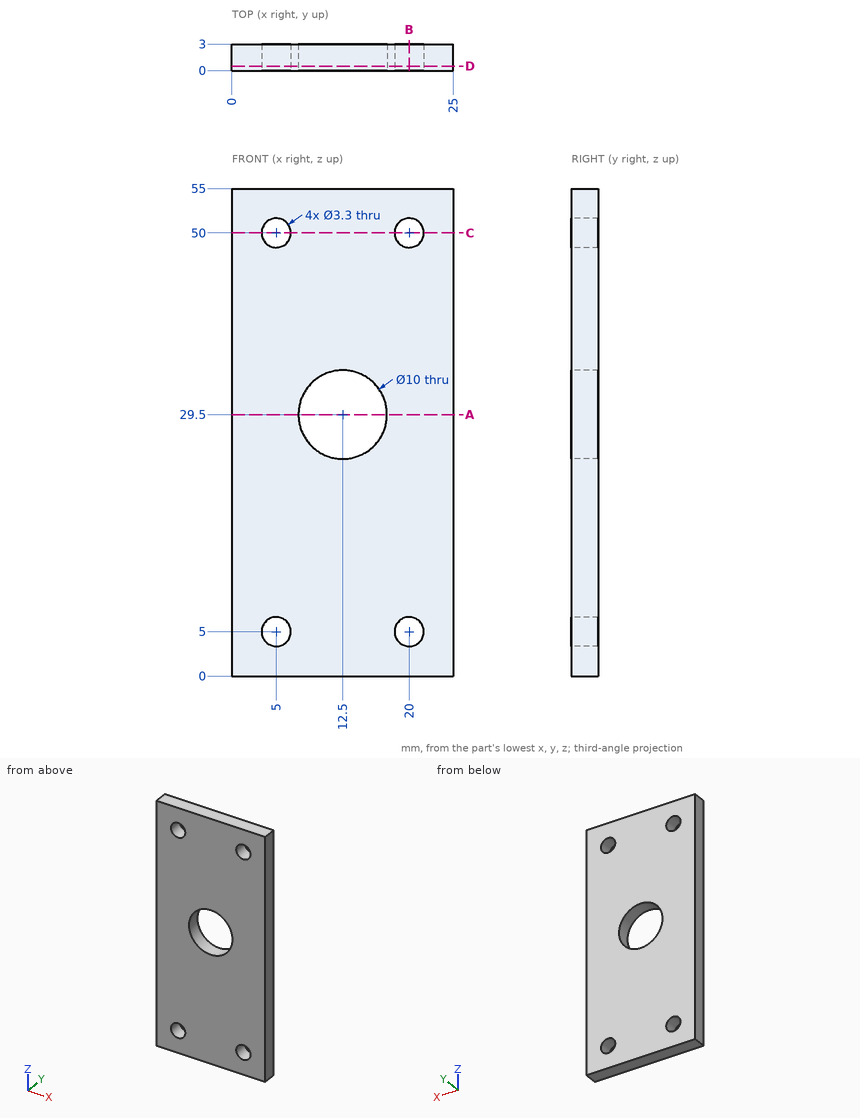
Geometry: see drawing. Coordinates: mm, zero at the bounding-box minimum. Give positions to 0.01 mm unless a question says otherwise; leave off trailing zeros. Loops run counter-clockwise (first coordinate to the right, second up) from the corner with the lowest first, then second, coordinate; pieces in that order, holes last. Notation, with made-up numbers: M 36.5,19 L 54.5,19 A19 ccw 54.5,48 Z; hole C -34,-31 d11. An arc over 180 degrees is marked long. Use one line per item in the form item = value.
1. Section query B-B, the plane x = 20. Return the cut outline in (y, z).
Numbers:
outline = M 0,0 L 3,0 L 3,3.35 L 0,3.35 Z; M 0,6.65 L 3,6.65 L 3,48.35 L 0,48.35 Z; M 0,51.65 L 3,51.65 L 3,55 L 0,55 Z
2. Section query C-C, the plane z = 50. Return the cut outline in (x, y).
Numbers:
outline = M 0,0 L 3.35,0 L 3.35,3 L 0,3 Z; M 6.65,0 L 18.35,0 L 18.35,3 L 6.65,3 Z; M 21.65,0 L 25,0 L 25,3 L 21.65,3 Z
3. First-contact query: pin 1 (3 mm diameter, centred on x = 20, z = 50, fed in from +Y). Flat tip, straight axial feed; report the tip coordinate or a pass-through.
Numbers:
pin_1 = through
4. Line query: L1, parallel to X at y = 1.8, z = 5; L2, parallel to Z at x = 20, y = 1.25; L3, parallel to X at y = 1.4, z = 6. Output: solid intervals per line, ascending.
Numbers:
L1 = 0 to 3.35, 6.65 to 18.35, 21.65 to 25
L2 = 0 to 3.35, 6.65 to 48.35, 51.65 to 55
L3 = 0 to 3.69, 6.31 to 18.69, 21.31 to 25
5. Section query D-D, the plane y = 0.5. Return the cut outline in (x, z).
Numbers:
outline = M 0,0 L 25,0 L 25,55 L 0,55 Z; hole C 5,5 d3.3; hole C 5,50 d3.3; hole C 12.5,29.5 d10; hole C 20,5 d3.3; hole C 20,50 d3.3
6. Section query A-A, the plane z = 29.5. Return the cut outline in (x, y).
Numbers:
outline = M 0,0 L 7.5,0 L 7.5,3 L 0,3 Z; M 17.5,0 L 25,0 L 25,3 L 17.5,3 Z
